Source: CAD feature listing. Evaluate the final solid. Frame: model axes, mm. A direction names the side the tool comes from. Coordinates: 2 decimals unless noted, no trailing zeros. Write each loop counter-clockwise with the first axis right and the second up, starting at its lowest first coordinate (ties: lowest second). Pieces come first, ordered by that corner, then holes. Notation, with made-up numbers: (10.5, 52) -> (47.5, 52) arc R25 cw to (47.5, 77) -> close; hole circle Ø1 at (56, 3). An arc over 180 degrees is marked (long way). One line per item, written item: value. Start each with the question number.
1. Mould query, pull axis X, two halves, no side actions, for faces 1 (the flat face through (100, 6.35, 122)), 2 (the flat face through (122, 58.928, 51)), 3 (the flat face through (203.2, 33, 55)). Classes: released by +X, released by -X, zero draft, split by the parting line, or undercut.
2. Section query C-C, the plane x = 140. Output: boundary loops of the cut face in (y, z), and give its area (3 significant figures).
3. First-contact query: P1, Ø1, axis at x = 28.5, z = 73, coming from the +Y side; P2, Ø24, axis at y = 69.5, z = 31, coming from the +X side; P3, Ø3, axis at y = 60.5, z = 24.5, coming from the +X side; P4, Ø4, axis at y = 82, z = 18, coming from the -X side. Flat tips, straight axial feed; report the tip coordinate or a pass-through.
4. Access query for faces 4 (the flat face through (107.696, 61, 79)), 5 (the flat face through (103, 47, 101.6)), 6 (the flat face through (195.199, 66, 75)). Directions: +Z, -Z, +X, -X, +Y, -Y. A direction counts if a zero-diameter tool reaches every point of the face in a straight line with its end or side. Return the directions, or none.
5. Line query: line 1 (Z direction, x = 77, y = 44); line 2 (Z direction, x = 42, y = 79); line 3 (Z direction, x = 51, y = 82). Output: solid intervals per line, ascending.
6. Section query B-B, the plane y = 29.5. Output: boundary loops of the cut face in (x, z).
from build123d import *

# Parameters (mm, degrees)
BOSS_EXTRUDE1_DEPTH = 88.89999999999999
SKETCH2_R           = 29.97200000000001
CUT_EXTRUDE1_DEPTH  = 203.2
CUT_EXTRUDE2_DEPTH  = 8.001
SKETCH4_W           = 59.943999999999946
SKETCH4_H           = 29.972
CUT_EXTRUDE3_DEPTH  = 27.94
SKETCH5_R           = 38.417500000000004
CUT_EXTRUDE4_DEPTH  = 107.696
CUT_EXTRUDE5_DEPTH  = 5.08
SKETCH7_W           = 203.19999999999996
SKETCH7_H           = 6.349999999999999
BOSS_EXTRUDE2_DEPTH = 38.1
FILLET1_R           = 2.54


with BuildPart() as part:
    # Sketch1 → Boss-Extrude1 (new body)
    with BuildSketch(Plane(origin=(0, 0, 0), x_dir=(1, 0, 0), z_dir=(0, 1, 0))):
        Polygon((0, 0), (203.2, 0), (203.2, -101.6), (1.244e-14, -101.6), align=None)
    extrude(amount=BOSS_EXTRUDE1_DEPTH)

    # Sketch2 → Cut-Extrude1 (cut)
    with BuildSketch(Plane(origin=(203.2, 0, 0), x_dir=(-2.2e-16, 0, -1), z_dir=(1, 0, -2.2e-16))):
        with Locations((-50.8, 88.89999999999999)):
            Circle(SKETCH2_R)
    extrude(amount=-CUT_EXTRUDE1_DEPTH, mode=Mode.SUBTRACT)

    # Sketch3 → Cut-Extrude2 (cut)
    with BuildSketch(Plane(origin=(203.2, 0, 0), x_dir=(-2.2e-16, 0, -1), z_dir=(1, 0, -2.2e-16))):
        Polygon((-20.82800000000002, 118.87199999999997), (-80.77199999999996, 118.87199999999996), (-80.77199999999996, 58.928000000000004), (-20.828000000000007, 58.928000000000004), align=None)
    extrude(amount=-CUT_EXTRUDE2_DEPTH, mode=Mode.SUBTRACT)

    # Sketch4 → Cut-Extrude3 (cut)
    with BuildSketch(Plane(origin=(135.636, 0, 0), x_dir=(-2.2e-16, 0, -1), z_dir=(1, 0, -2.2e-16))):
        with Locations((-50.800000000000004, 73.914)):
            Rectangle(SKETCH4_W, SKETCH4_H)
    extrude(amount=-CUT_EXTRUDE3_DEPTH, mode=Mode.SUBTRACT)

    # Sketch5 → Cut-Extrude4 (cut)
    with BuildSketch(Plane.ZY):
        with Locations((50.8, 88.89999999999999)):
            Circle(SKETCH5_R)
    extrude(amount=-CUT_EXTRUDE4_DEPTH, mode=Mode.SUBTRACT)

    # Sketch6 → Cut-Extrude5 (cut)
    with BuildSketch(Plane(origin=(0, 58.928000000000004, 0), x_dir=(1, 0, 0), z_dir=(0, 1, 0))):
        with BuildLine():
            ThreePointArc((121.66599999999983, -34.29000000000002), (114.68100000000004, -41.275000000000006), (121.66599999999983, -48.25999999999999))
            Line((121.66600000000003, -48.25999999999999), (121.66600000000003, -34.29000000000002))
        make_face()
        with BuildLine():
            Line((121.66600000000003, -34.29000000000002), (121.66600000000003, -48.25999999999999))
            ThreePointArc((121.66599999999983, -48.25999999999999), (126.60514086658797, -46.214140866588096), (128.651, -41.275000000000006))
            ThreePointArc((128.651, -41.275000000000006), (126.60514086658797, -36.335859133411915), (121.66599999999983, -34.29000000000002))
        make_face()
    extrude(amount=-CUT_EXTRUDE5_DEPTH, mode=Mode.SUBTRACT)

    # Sketch7 → Boss-Extrude2 (add)
    with BuildSketch(Plane.XY.offset(101.6)):
        with Locations((101.59999999999998, 3.1749999999999994)):
            Rectangle(SKETCH7_W, SKETCH7_H)
    extrude(amount=BOSS_EXTRUDE2_DEPTH)

    # Fillet1
    fillet1_edges = [part.edges().sort_by_distance(p)[0] for p in [
        (101.6, 6.35, 101.6),
        (0, 6.35, 120.64999999999999),
        (203.2, 6.35, 120.64999999999999),
        (0, 44.449999999999996, 0),
        (1.168e-14, 88.89999999999999, 95.40875),
        (1.244e-14, 47.625, 101.6),
        (101.6, 88.89999999999999, 0),
        (203.2, 44.449999999999996, 0),
        (203.2, 88.89999999999999, 10.413999999999994),
        (203.2, 88.89999999999999, 91.186),
        (101.6, 88.89999999999999, 101.6),
        (203.2, 47.625, 101.6),
    ]]
    fillet(fillet1_edges, radius=FILLET1_R)


solid = part.part
Computed values:
1. face 1: zero draft
1. face 2: undercut
1. face 3: released by +X
2. outline: (0, 0) -> (86.36, 0) arc R2.54 ccw to (88.9, 2.54) -> (88.9, 20.83) arc R29.97 cw to (88.9, 80.77) -> (88.9, 99.06) arc R2.54 ccw to (86.36, 101.6) -> (8.89, 101.6) arc R2.54 cw to (6.35, 104.14) -> (6.35, 139.7) -> (0, 139.7) -> close
2. area: 7,860 mm²
3. P1: stops at y = 57.91
3. P2: stops at x = 203.2
3. P3: stops at x = 195.2
3. P4: stops at x = 107.7
4. face 4: +Y
4. face 5: +Z, +X, -X, +Y
4. face 6: +X, +Y
5. line 1: z = 0 to 101.6
5. line 2: z = 0 to 13.68, 87.92 to 101.6
5. line 3: z = 0 to 13.01, 88.59 to 101.6
6. outline: (0, 2.54) arc R2.54 ccw to (2.54, 0) -> (200.66, 0) arc R2.54 ccw to (203.2, 2.54) -> (203.2, 99.06) arc R2.54 ccw to (200.66, 101.6) -> (2.54, 101.6) arc R2.54 ccw to (0, 99.06) -> close
